from build123d import *

# Parameters (mm, degrees)
CROQUIS2_OUTSIDE_W    = 35.33
CROQUIS2_OUTSIDE_H    = 35.33
CORTAR_EXTRUIR2_DEPTH = 40


with BuildPart() as part:
    # Croquis1 → Revolución1 (revolve)
    with BuildSketch(Plane(origin=(0, 0, 0), x_dir=(1, 0, 0), z_dir=(0, 1, 0))):
        Polygon((5, 26.679286354), (10, 26.679286354), (10, 24.679286354), (9, 24.679286354), (9, 21.679286354), (10, 21.679286354), (10, 20.679286354), (12, 18.574849316), (12, 8.21549426), (7.464345365, 5.21549426), (7.464345365, 4.439385), (8.179362134, 3.961906928), (8.179362134, -4.011582493), (6.20010654, -5.320713646), (5, -5.320713646), align=None)
    revolve(axis=Axis((0, 0, -34.95637535), (0, 0, 1)))

    # Croquis2 outside → Cortar-Extruir2 (cut)
    with BuildSketch(Plane.XY):
        Rectangle(CROQUIS2_OUTSIDE_W, CROQUIS2_OUTSIDE_H)
        Polygon((12, 0), (6, 10.392304845), (-6, 10.392304845), (-12, 0), (-6, -10.392304845), (6, -10.392304845), align=None, mode=Mode.SUBTRACT)
    extrude(amount=-CORTAR_EXTRUIR2_DEPTH, mode=Mode.SUBTRACT)


solid = part.part
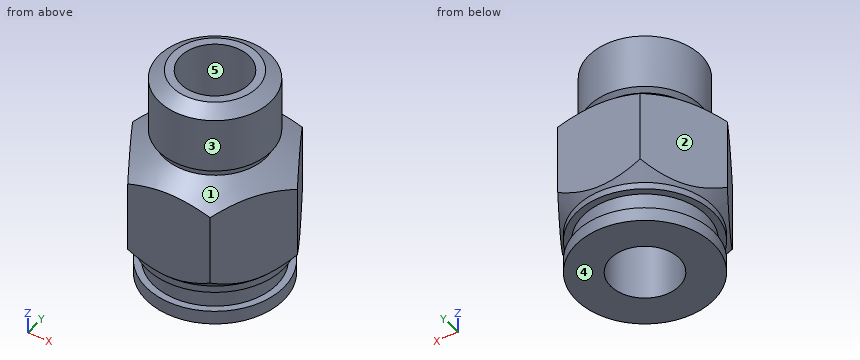
CAD build for the part. Positions are in the model's coordinates, mm. Face numbers are marked on the shaded views. A direction names the side the tool comes from. Round coordinates to 2 decimals unless told otherwise and drop trailing zeros. Order: outer loops, then holes, each group sorted by start corner. A loop starts at its lowest first (then second) coordinate and runs counter-clockwise, first axis right, second up. Notation, with made-up numbers: M 89,88 L 138,88 A16 cw 138,112 Z; hole C 1,87 d9. An arc over 180 degrees is marked long. Use one line per item in the form item = value.
Q1. Saw through at B-B on z = -9. Give the cut face in (x, y).
Recorded:
outline = M -12,0 L -6,-10.39 L 6,-10.39 L 12,0 L 6,10.39 L -6,10.39 Z; hole C 0,0 d10
Q2. Which spindle directions (+Z, -Z, +X, -X, +Y, -Y) get a long thin tool onto all of the face, cutting with end or side? Do the marked faces 1 and 2. Say none if no direction does.
Recorded:
face_1 = none
face_2 = +Z, -Z, -X, +Y
Q3. Two-plate mould, pull along X, no slides. Class the marked faces 3, 4 and 5: +X half, -X half, draft (parallel to the pull), parting line (faces both ways), or undercut.
Recorded:
face_3 = parting line
face_4 = draft
face_5 = undercut
Q4. Probe L1, parallel to Y at x = 0, z = -13; L2, parallel to Y at x = 0, z = -3; L3, parallel to X at y = -3.75, z = -7.5. List the from-to ranges inside material, lowest first.
Recorded:
L1 = -10.39 to -5, 5 to 10.39
L2 = -8.18 to -5, 5 to 8.18
L3 = -9.83 to -3.31, 3.31 to 9.83
Q5. Saw through at C-C on z = -22.5. Give the cut face in (x, y), then the cut area to 3 significant figures.
Recorded:
outline = C 0,0 d18; hole C 0,0 d10
area = 176 mm^2
Q6. Flat gauge pins, fed straight in: P1, Ø6, axis at y = 5.5, z = -1, coming from the +X side; P2, Ø6, axis at x = 8, y = 6, coming from the +Z side. Where does each tip first touch, or does it go through?
Recorded:
P1 = 7.79
P2 = 4.79
